Check sheet for the modelled part. Datum: model origin and axes. Units: mm. A direction names the side the tool comes from. Round coordinates to 2 decimals unless told otherwise and drop trailing zeros. Write each loop counter-clockwise with the first axis right and the second up, starting at its lowest first coordinate (ties: lowest second). Pieces come first, ordered by that corner, then holes.
Item 1: Go/stop test with flat-tipped pins: pin 1 Ø8 at (x, y) = (6, -7) entering from -Z; pin 2 Ø1 at (x, z) = (6.5, 76) entering from +Y; pin 3 Ø0.6 at (y, z) = (-8, 72) entering from +X; pin 4 Ø4 at (x, z) = (2, 39) entering from -Y. Record where each tip stops, or that it passes through.
Item 2: Cross-section at D-D on z = 27. Count the separate pieces of the cut face and the enclosed holes in it, plus the area to 3 significant figures.
Item 3: Cross-section at A-A on x = 4.75. Enter the section's corners in (y, z).
Item 4: Release check for a two-part mould opening along X. For faces 1 (the cylindrical face through (17.41, -26.61, 49.3)), 2 (the flat face through (-11.842, -3, 49)), 3 (the flat face through (14, -4.074, 49)) record: +X half, -X half, draft (parallel to the pull), parting line (faces both ways), or undercut.
Item 5: Cross-section at B-B on y = -10.75. Enter the section's corners in (x, z), plus the area to 3 significant figures.
Item 6: Cross-section at C-C on x = 10. Enter the section's corners in (y, z), plus the area to 3 significant figures.
Item 7: Tool access check on faces 4 (the flat face through (-11.842, -21, 49)), 5 (the flat face through (9, -25.124, 49)). Record the directions out of +Z, -Z, +X, -X, +Y, -Y that give a thin tool (end or side, any length) a straight path to the whole face; none if there is none.
Item 8: Material ranges on line 1 (Y direction, x = -7, z = 15); line 2 (Y direction, x = -1, z = 62.5); line 3 (X direction, y = 0, z = 43.5), recorded low to high.
from build123d import *

# Parameters (mm, degrees)
SKETCH_1_R      = 3.4
EXTRUDE_1_DEPTH = 100


with BuildPart() as part:
    # 草图1 → 凸台-拉伸1 (new body)
    with BuildSketch(Plane.XY):
        with BuildLine():
            Line((8.957955872, -8.080050324), (12.963590791, -4.074415406))
            Line((12.963590791, -4.074415406), (15.657955872, -4.074415406))
            ThreePointArc((15.657955872, -4.074415406), (15.870087906, -4.162283371), (15.957955872, -4.374415406))
            Line((15.957955872, -4.374415406), (15.957955872, -7.924415406))
            ThreePointArc((15.957955872, -7.924415406), (16.045823838, -8.13654744), (16.257955872, -8.224415406))
            Line((16.257955872, -8.224415406), (17.157955872, -8.224415406))
            Line((17.157955872, -8.224415406), (17.157955872, -7.424415406))
            ThreePointArc((17.157955872, -7.424415406), (17.216534516, -7.28299405), (17.357955872, -7.224415406))
            Line((17.357955872, -7.224415406), (18.157955872, -7.224415406))
            Line((18.157955872, -7.224415406), (18.157955872, 0.175584594))
            ThreePointArc((18.157955872, 0.175584594), (17.425722825, 1.943351547), (15.657955872, 2.675584594))
            Line((15.657955872, 2.675584594), (8.257955872, 2.675584594))
            Line((8.257955872, 2.675584594), (8.257955872, 1.875584594))
            ThreePointArc((8.257955872, 1.875584594), (8.199377228, 1.734163238), (8.057955872, 1.675584594))
            Line((8.057955872, 1.675584594), (7.257955872, 1.675584594))
            Line((7.257955872, 1.675584594), (7.257955872, 0.775584594))
            ThreePointArc((7.257955872, 0.775584594), (7.345823838, 0.56345256), (7.557955872, 0.475584594))
            Line((7.557955872, 0.475584594), (11.107955872, 0.475584594))
            ThreePointArc((11.107955872, 0.475584594), (11.320087906, 0.387716629), (11.407955872, 0.175584594))
            Line((11.407955872, 0.175584594), (11.407955872, -2.518780487))
            Line((11.407955872, -2.518780487), (7.402320953, -6.524415406))
            Line((7.402320953, -6.524415406), (-1.086409209, -6.524415406))
            Line((-1.086409209, -6.524415406), (-5.092044128, -2.518780487))
            Line((-5.092044128, -2.518780487), (-5.092044128, 0.175584594))
            ThreePointArc((-5.092044128, 0.175584594), (-5.004176162, 0.387716629), (-4.792044128, 0.475584594))
            Line((-4.792044128, 0.475584594), (-1.242044128, 0.475584594))
            ThreePointArc((-1.242044128, 0.475584594), (-1.029912094, 0.56345256), (-0.942044128, 0.775584594))
            Line((-0.942044128, 0.775584594), (-0.942044128, 1.675584594))
            Line((-0.942044128, 1.675584594), (-1.742044128, 1.675584594))
            ThreePointArc((-1.742044128, 1.675584594), (-1.883465484, 1.734163238), (-1.942044128, 1.875584594))
            Line((-1.942044128, 1.875584594), (-1.942044128, 2.675584594))
            Line((-1.942044128, 2.675584594), (-9.342044128, 2.675584594))
            ThreePointArc((-9.342044128, 2.675584594), (-11.109811081, 1.943351547), (-11.842044128, 0.175584594))
            Line((-11.842044128, 0.175584594), (-11.842044128, -7.224415406))
            Line((-11.842044128, -7.224415406), (-11.042044128, -7.224415406))
            ThreePointArc((-11.042044128, -7.224415406), (-10.900622772, -7.28299405), (-10.842044128, -7.424415406))
            Line((-10.842044128, -7.424415406), (-10.842044128, -8.224415406))
            Line((-10.842044128, -8.224415406), (-9.942044128, -8.224415406))
            ThreePointArc((-9.942044128, -8.224415406), (-9.729912094, -8.13654744), (-9.642044128, -7.924415406))
            Line((-9.642044128, -7.924415406), (-9.642044128, -4.374415406))
            ThreePointArc((-9.642044128, -4.374415406), (-9.554176162, -4.162283371), (-9.342044128, -4.074415406))
            Line((-9.342044128, -4.074415406), (-6.647679047, -4.074415406))
            Line((-6.647679047, -4.074415406), (-2.642044128, -8.080050324))
            Line((-2.642044128, -8.080050324), (-2.642044128, -16.568780487))
            Line((-2.642044128, -16.568780487), (-6.647679047, -20.574415406))
            Line((-6.647679047, -20.574415406), (-9.342044128, -20.574415406))
            ThreePointArc((-9.342044128, -20.574415406), (-9.554176162, -20.48654744), (-9.642044128, -20.274415406))
            Line((-9.642044128, -20.274415406), (-9.642044128, -16.724415406))
            ThreePointArc((-9.642044128, -16.724415406), (-9.729912094, -16.512283371), (-9.942044128, -16.424415406))
            Line((-9.942044128, -16.424415406), (-10.842044128, -16.424415406))
            Line((-10.842044128, -16.424415406), (-10.842044128, -17.224415406))
            ThreePointArc((-10.842044128, -17.224415406), (-10.900622772, -17.365836762), (-11.042044128, -17.424415406))
            Line((-11.042044128, -17.424415406), (-11.842044128, -17.424415406))
            Line((-11.842044128, -17.424415406), (-11.842044128, -24.824415406))
            ThreePointArc((-11.842044128, -24.824415406), (-11.109811081, -26.592182359), (-9.342044128, -27.324415406))
            Line((-9.342044128, -27.324415406), (-1.942044128, -27.324415406))
            Line((-1.942044128, -27.324415406), (-1.942044128, -26.524415406))
            ThreePointArc((-1.942044128, -26.524415406), (-1.883465484, -26.38299405), (-1.742044128, -26.324415406))
            Line((-1.742044128, -26.324415406), (-0.942044128, -26.324415406))
            Line((-0.942044128, -26.324415406), (-0.942044128, -25.424415406))
            ThreePointArc((-0.942044128, -25.424415406), (-1.029912094, -25.212283371), (-1.242044128, -25.124415406))
            Line((-1.242044128, -25.124415406), (-4.792044128, -25.124415406))
            ThreePointArc((-4.792044128, -25.124415406), (-5.004176162, -25.03654744), (-5.092044128, -24.824415406))
            Line((-5.092044128, -24.824415406), (-5.092044128, -22.130050324))
            Line((-5.092044128, -22.130050324), (-1.086409209, -18.124415406))
            Line((-1.086409209, -18.124415406), (7.402320953, -18.124415406))
            Line((7.402320953, -18.124415406), (11.407955872, -22.130050324))
            Line((11.407955872, -22.130050324), (11.407955872, -24.824415406))
            ThreePointArc((11.407955872, -24.824415406), (11.320087906, -25.03654744), (11.107955872, -25.124415406))
            Line((11.107955872, -25.124415406), (7.557955872, -25.124415406))
            ThreePointArc((7.557955872, -25.124415406), (7.345823838, -25.212283371), (7.257955872, -25.424415406))
            Line((7.257955872, -25.424415406), (7.257955872, -26.324415406))
            Line((7.257955872, -26.324415406), (8.057955872, -26.324415406))
            ThreePointArc((8.057955872, -26.324415406), (8.199377228, -26.38299405), (8.257955872, -26.524415406))
            Line((8.257955872, -26.524415406), (8.257955872, -27.324415406))
            Line((8.257955872, -27.324415406), (15.657955872, -27.324415406))
            ThreePointArc((15.657955872, -27.324415406), (17.425722825, -26.592182359), (18.157955872, -24.824415406))
            Line((18.157955872, -24.824415406), (18.157955872, -17.424415406))
            Line((18.157955872, -17.424415406), (17.357955872, -17.424415406))
            ThreePointArc((17.357955872, -17.424415406), (17.216534516, -17.365836762), (17.157955872, -17.224415406))
            Line((17.157955872, -17.224415406), (17.157955872, -16.424415406))
            Line((17.157955872, -16.424415406), (16.257955872, -16.424415406))
            ThreePointArc((16.257955872, -16.424415406), (16.045823838, -16.512283371), (15.957955872, -16.724415406))
            Line((15.957955872, -16.724415406), (15.957955872, -20.274415406))
            ThreePointArc((15.957955872, -20.274415406), (15.870087906, -20.48654744), (15.657955872, -20.574415406))
            Line((15.657955872, -20.574415406), (12.963590791, -20.574415406))
            Line((12.963590791, -20.574415406), (8.957955872, -16.568780487))
            Line((8.957955872, -16.568780487), (8.957955872, -8.080050324))
        make_face()
        with Locations((3.157955872, -12.324415406)):
            Circle(SKETCH_1_R, mode=Mode.SUBTRACT)
        with BuildLine():
            Line((13.907955872, -22.074415406), (15.657955872, -22.074415406))
            ThreePointArc((15.657955872, -22.074415406), (16.365062653, -22.367308625), (16.657955872, -23.074415406))
            Line((16.657955872, -23.074415406), (16.657955872, -24.824415406))
            ThreePointArc((16.657955872, -24.824415406), (16.365062653, -25.531522187), (15.657955872, -25.824415406))
            Line((15.657955872, -25.824415406), (13.907955872, -25.824415406))
            ThreePointArc((13.907955872, -25.824415406), (13.200849091, -25.531522187), (12.907955872, -24.824415406))
            Line((12.907955872, -24.824415406), (12.907955872, -23.074415406))
            ThreePointArc((12.907955872, -23.074415406), (13.200849091, -22.367308625), (13.907955872, -22.074415406))
        make_face(mode=Mode.SUBTRACT)
        with BuildLine():
            Line((12.907955872, -1.574415406), (12.907955872, 0.175584594))
            ThreePointArc((12.907955872, 0.175584594), (13.200849091, 0.882691375), (13.907955872, 1.175584594))
            Line((13.907955872, 1.175584594), (15.657955872, 1.175584594))
            ThreePointArc((15.657955872, 1.175584594), (16.365062653, 0.882691375), (16.657955872, 0.175584594))
            Line((16.657955872, 0.175584594), (16.657955872, -1.574415406))
            ThreePointArc((16.657955872, -1.574415406), (16.365062653, -2.281522187), (15.657955872, -2.574415406))
            Line((15.657955872, -2.574415406), (13.907955872, -2.574415406))
            ThreePointArc((13.907955872, -2.574415406), (13.200849091, -2.281522187), (12.907955872, -1.574415406))
        make_face(mode=Mode.SUBTRACT)
        with BuildLine():
            Line((-6.592044128, -23.074415406), (-6.592044128, -24.824415406))
            ThreePointArc((-6.592044128, -24.824415406), (-6.884937347, -25.531522187), (-7.592044128, -25.824415406))
            Line((-7.592044128, -25.824415406), (-9.342044128, -25.824415406))
            ThreePointArc((-9.342044128, -25.824415406), (-10.049150909, -25.531522187), (-10.342044128, -24.824415406))
            Line((-10.342044128, -24.824415406), (-10.342044128, -23.074415406))
            ThreePointArc((-10.342044128, -23.074415406), (-10.049150909, -22.367308625), (-9.342044128, -22.074415406))
            Line((-9.342044128, -22.074415406), (-7.592044128, -22.074415406))
            ThreePointArc((-7.592044128, -22.074415406), (-6.884937347, -22.367308625), (-6.592044128, -23.074415406))
        make_face(mode=Mode.SUBTRACT)
        with BuildLine():
            Line((-7.592044128, -2.574415406), (-9.342044128, -2.574415406))
            ThreePointArc((-9.342044128, -2.574415406), (-10.049150909, -2.281522187), (-10.342044128, -1.574415406))
            Line((-10.342044128, -1.574415406), (-10.342044128, 0.175584594))
            ThreePointArc((-10.342044128, 0.175584594), (-10.049150909, 0.882691375), (-9.342044128, 1.175584594))
            Line((-9.342044128, 1.175584594), (-7.592044128, 1.175584594))
            ThreePointArc((-7.592044128, 1.175584594), (-6.884937347, 0.882691375), (-6.592044128, 0.175584594))
            Line((-6.592044128, 0.175584594), (-6.592044128, -1.574415406))
            ThreePointArc((-6.592044128, -1.574415406), (-6.884937347, -2.281522187), (-7.592044128, -2.574415406))
        make_face(mode=Mode.SUBTRACT)
    extrude(amount=EXTRUDE_1_DEPTH)


solid = part.part
Response values:
1. pin 1: stops at z = 0
1. pin 2: stops at y = -6.52
1. pin 3: stops at x = 17.16
1. pin 4: stops at y = -18.12
2. separate pieces: 1
2. enclosed holes: 5
2. area: 328 mm2
3. outline: (-18.12, 0) - (-15.33, 0) - (-15.33, 100) - (-18.12, 100) - close; (-9.32, 0) - (-6.52, 0) - (-6.52, 100) - (-9.32, 100) - close
4. face 1: +X half
4. face 2: -X half
4. face 3: undercut
5. outline: (-2.64, 0) - (0.14, 0) - (0.14, 100) - (-2.64, 100) - close; (6.17, 0) - (8.96, 0) - (8.96, 100) - (6.17, 100) - close
5. area: 557 mm2
6. outline: (-27.32, 0) - (-25.12, 0) - (-25.12, 100) - (-27.32, 100) - close; (-20.72, 0) - (-17.61, 0) - (-17.61, 100) - (-20.72, 100) - close; (-7.04, 0) - (-3.93, 0) - (-3.93, 100) - (-7.04, 100) - close; (0.48, 0) - (2.68, 0) - (2.68, 100) - (0.48, 100) - close
6. area: 1,060 mm2
7. face 4: +Z, -Z, -X, +Y, -Y
7. face 5: +Z, -Z
8. line 1: y = -27.32 to -25.63, -22.27 to -20.57, -4.07 to -2.38, 0.98 to 2.68
8. line 2: y = -26.32 to -25.25, -18.12 to -6.52, 0.6 to 1.68
8. line 3: x = -11.84 to -10.34, -6.59 to -5.09, 11.41 to 12.91, 16.66 to 18.16
